Can you work these out from the model? Positions are in its coordinate system, mm. Face numbers are marked on the shaded views. A direction names the side the tool comes from. Give positions to 0.01 mm unless a question says otherwise; leave off trailing zeros. Order: outer loops, then holes, each group sorted by start corner. A loop starts at its lowest first (then second) coordinate and runs counter-clockwise, first axis right, second up.
Item 1: I want a section at C-C, the plane x = 0. Write out the boundary of the cut face in (y, z) (1 decimal).
Item 2: I want a section at A-A, the plane y = 5. Write out the boundary of the cut face in (x, z) (3 decimals), then the cut area to 3 significant figures.
Item 3: If we mould it in two halves opening along Y, with no side actions, what happens to the marked faces 3, 4 and 5? For each: +Y half, -Y half, draft (parallel to the pull), parting line (faces both ways), or undercut.
Item 4: I want a section at B-B, the plane z = 8.5. Write out the boundary of the cut face in (x, y) (3 decimals), then the cut area to 3 significant figures.
Item 5: I'm going to push flat-ended pins straight in: pin 1 Ø6.5 at (x, y) = (-12, 11.5) entering from -Z; pin 2 Ø1 at (y, z) = (-0.5, 8) entering from -X. Where does each tip first touch, or does it pass through?
Item 6: If I drill on line 1 along X through (y, z) = (7.25, 11.25) (3 decimals); line 2 along X through (y, z) = (4, 10) (3 decimals); line 3 along Y through (x, z) = (0, 4.25) (1 decimal), over which ranges is the centre line in solid material (lowest first)?
Item 7: I want a section at D-D, the plane y = 0. Write out the boundary of the cut face in (x, z) (3 decimals).
Item 8: Which directions (+Z, -Z, +X, -X, +Y, -Y) give clear straight access to the entire face, cutting with the end or side of a thin tool? Please do the marked faces 1 and 2.
```python
from build123d import *

# Parameters (mm, degrees)
F1_R     = 2.3375
F2_DEPTH = 7.5
F1_R_2   = 2.675
F4_DEPTH = 5
F5_R     = 5
F7_DEPTH = 2.75


# Not quite as in the source:
# - a feature names something its author has since deleted; it is built from what else it names


with BuildPart() as f2:
    # F1 (on Top) → F2 (new body)
    with BuildSketch(Plane.XY):
        with Locations((0, 19.305)):
            Circle(F1_R)
    extrude(amount=F2_DEPTH)



with BuildPart() as f2b:
    # F1 (on Top) → F2, piece 2 (new body)
    with BuildSketch(Plane.XY):
        Circle(F1_R_2)
    extrude(amount=F2_DEPTH)


with BuildPart() as f2_1:
    add(f2.part)

    add(f2b.part)  # F4 merges F2b
    # F3 (on face) → F4 (join)
    with BuildSketch(Plane.XY.offset(7.5)):
        with BuildLine():
            Line((0, 21.6425), (0, 22.805))
            Line((0, 22.805), (-10.675, 22.805))
            Line((-10.675, 22.805), (-10.675, 20.005))
            ThreePointArc((-10.675, 20.005), (-9.472918472, 19.507081528), (-8.975, 18.305))
            Line((-8.975, 18.305), (-8.975, 1))
            ThreePointArc((-8.975, 1), (-9.472918472, -0.202081528), (-10.675, -0.7))
            Line((-10.675, -0.7), (-10.675, -3.5))
            Line((-10.675, -3.5), (0, -3.5))
            Line((0, -3.5), (0, 16.9675))
            ThreePointArc((0, 16.9675), (-2.3375, 19.305), (0, 21.6425))
        make_face()
        with BuildLine():
            Line((10.675, 22.805), (0, 22.805))
            Line((0, 22.805), (0, 21.6425))
            ThreePointArc((0, 21.6425), (1.652862101, 20.957862101), (2.3375, 19.305))
            ThreePointArc((2.3375, 19.305), (1.652862101, 17.652137899), (0, 16.9675))
            Line((0, 16.9675), (0, -3.5))
            Line((0, -3.5), (10.675, -3.5))
            Line((10.675, -3.5), (10.675, -0.7))
            ThreePointArc((10.675, -0.7), (9.472918472, -0.202081528), (8.975, 1))
            Line((8.975, 1), (8.975, 18.305))
            ThreePointArc((8.975, 18.305), (9.472918472, 19.507081528), (10.675, 20.005))
            Line((10.675, 20.005), (10.675, 22.805))
        make_face()
        with BuildLine():
            Line((0, 16.9675), (0, 21.6425))
            ThreePointArc((0, 21.6425), (-2.3375, 19.305), (0, 16.9675))
        make_face()
        with BuildLine():
            ThreePointArc((2.3375, 19.305), (1.652862101, 20.957862101), (0, 21.6425))
            Line((0, 21.6425), (0, 16.9675))
            ThreePointArc((0, 16.9675), (1.652862101, 17.652137899), (2.3375, 19.305))
        make_face()
        with BuildLine():
            Line((-10.675, 20.005), (-10.675, 22.805))
            Line((-10.675, 22.805), (-18.175, 22.805))
            Line((-18.175, 22.805), (-18.175, -3.5))
            Line((-18.175, -3.5), (-10.675, -3.5))
            Line((-10.675, -3.5), (-10.675, -0.7))
            ThreePointArc((-10.675, -0.7), (-11.877081528, -0.202081528), (-12.375, 1))
            Line((-12.375, 1), (-12.375, 18.305))
            ThreePointArc((-12.375, 18.305), (-11.877081528, 19.507081528), (-10.675, 20.005))
        make_face()
        with BuildLine():
            Line((18.175, 22.805), (10.675, 22.805))
            Line((10.675, 22.805), (10.675, 20.005))
            ThreePointArc((10.675, 20.005), (11.877081528, 19.507081528), (12.375, 18.305))
            Line((12.375, 18.305), (12.375, 1))
            ThreePointArc((12.375, 1), (11.877081528, -0.202081528), (10.675, -0.7))
            Line((10.675, -0.7), (10.675, -3.5))
            Line((10.675, -3.5), (18.175, -3.5))
            Line((18.175, -3.5), (18.175, 22.805))
        make_face()
    extrude(amount=F4_DEPTH)

    # F5
    f5_edges = [f2_1.edges().sort_by_distance(p)[0] for p in [
        (-18.175, 22.805, 10),
        (-18.175, -3.5, 10),
        (18.175, -3.5, 10),
        (18.175, 22.805, 10),
    ]]
    fillet(f5_edges, radius=F5_R)

    # F6 (on face) → F7 (cut)
    with BuildSketch(Plane(origin=(0, 0, 7.5), x_dir=(1, 0, 0), z_dir=(0, 0, -1))):
        Polygon((-7.675, 0.7320508076), (-10.675, 2.4641016151), (-13.675, 0.7320508076), (-13.675, -2.7320508076), (-10.675, -4.4641016151), (-7.675, -2.7320508076), align=None)
        Polygon((-7.675, -16.5729491924), (-7.675, -2.7320508076), (-10.675, -4.4641016151), (-13.675, -2.7320508076), (-13.675, -16.5729491924), (-10.675, -14.8408983849), align=None)
        Polygon((-7.675, -20.0370508076), (-7.675, -16.5729491924), (-10.675, -14.8408983849), (-13.675, -16.5729491924), (-13.675, -20.0370508076), (-10.675, -21.7691016151), align=None)
        Polygon((10.675, 2.4641016151), (7.675, 0.7320508076), (7.675, -2.7320508076), (10.675, -4.4641016151), (13.675, -2.7320508076), (13.675, 0.7320508076), align=None)
        Polygon((10.675, -4.4641016151), (7.675, -2.7320508076), (7.675, -16.5729491924), (10.675, -14.8408983849), (13.675, -16.5729491924), (13.675, -2.7320508076), align=None)
        Polygon((10.675, -14.8408983849), (7.675, -16.5729491924), (7.675, -20.0370508076), (10.675, -21.7691016151), (13.675, -20.0370508076), (13.675, -16.5729491924), align=None)
    extrude(amount=-F7_DEPTH, mode=Mode.SUBTRACT)


solid = f2_1.part
```
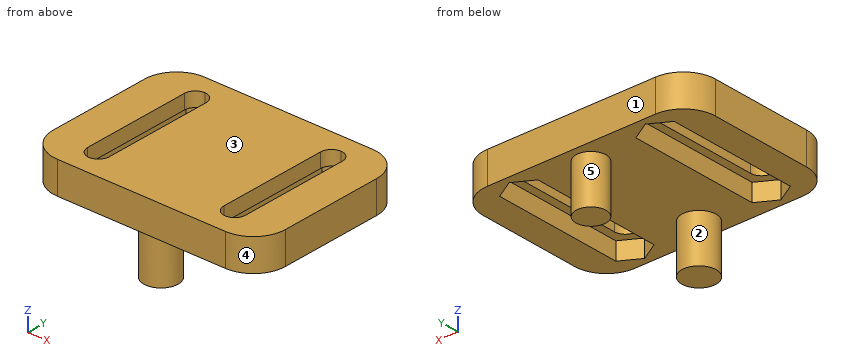
Results list:
1. outline: (-3.5, 7.5) - (-2.7, 7.5) - (-2.7, 0) - (2.7, 0) - (2.7, 7.5) - (17, 7.5) - (17, 0) - (21.6, 0) - (21.6, 7.5) - (22.8, 7.5) - (22.8, 12.5) - (-3.5, 12.5) - close
2. outline: (-18.175, 7.5) - (-13.675, 7.5) - (-13.675, 10.25) - (-12.375, 10.25) - (-12.375, 12.5) - (-18.175, 12.5) - close; (-8.975, 10.25) - (-7.675, 10.25) - (-7.675, 7.5) - (7.675, 7.5) - (7.675, 10.25) - (8.975, 10.25) - (8.975, 12.5) - (-8.975, 12.5) - close; (12.375, 10.25) - (13.675, 10.25) - (13.675, 7.5) - (18.175, 7.5) - (18.175, 12.5) - (12.375, 12.5) - close
2. area: 133 mm2
3. face 3: draft
3. face 4: -Y half
3. face 5: undercut
4. outline: (-18.175, 1.5) arc R5 ccw to (-13.175, -3.5) - (13.175, -3.5) arc R5 ccw to (18.175, 1.5) - (18.175, 17.805) arc R5 ccw to (13.175, 22.805) - (-13.175, 22.805) arc R5 ccw to (-18.175, 17.805) - close; hole (-13.675, -0.732) - (-10.675, -2.464) - (-7.675, -0.732) - (-7.675, 20.037) - (-10.675, 21.769) - (-13.675, 20.037) - close; hole (7.675, -0.732) - (10.675, -2.464) - (13.675, -0.732) - (13.675, 20.037) - (10.675, 21.769) - (7.675, 20.037) - close
4. area: 665 mm2
5. pin 1: stops at z = 7.5
5. pin 2: stops at x = -17.94
6. line 1: x = -18.175 to -12.375, -8.975 to 8.975, 12.375 to 18.175
6. line 2: x = -18.175 to -13.675, -7.675 to 7.675, 13.675 to 18.175
6. line 3: y = -2.7 to 2.7, 17 to 21.6
7. outline: (-17.945, 7.5) - (-13.675, 7.5) - (-13.675, 10.25) - (-12.05, 10.25) - (-12.05, 12.5) - (-17.945, 12.5) - close; (-9.3, 10.25) - (-7.675, 10.25) - (-7.675, 7.5) - (-2.675, 7.5) - (-2.675, 0) - (2.675, 0) - (2.675, 7.5) - (7.675, 7.5) - (7.675, 10.25) - (9.3, 10.25) - (9.3, 12.5) - (-9.3, 12.5) - close; (12.05, 10.25) - (13.675, 10.25) - (13.675, 7.5) - (17.945, 7.5) - (17.945, 12.5) - (12.05, 12.5) - close
8. face 1: +Z, -Z, +X, -X, +Y
8. face 2: -Z
